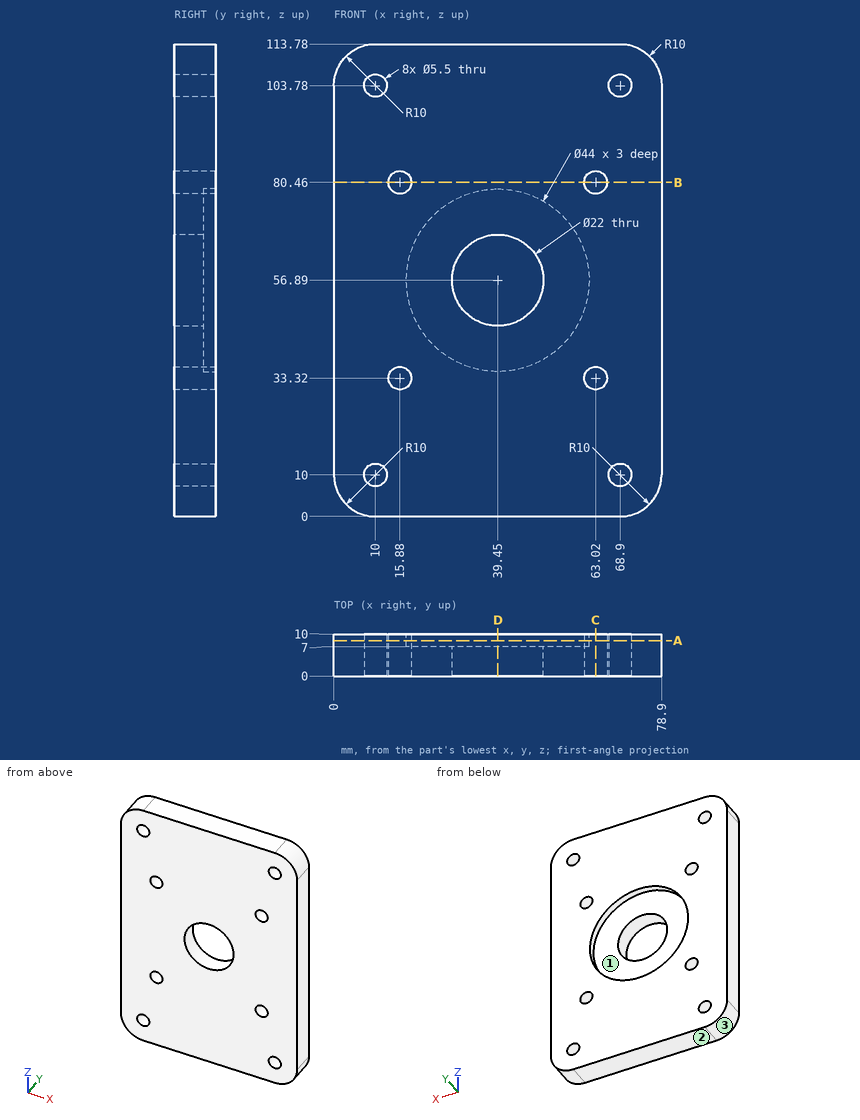
Job drawing, mm, ordinate dimensions from the low corner. One solid piece. Round coordinates to 2 decimals unless told otherwise and drop trailing zeros. Write each loop counter-clockwise with the first axis right and the second up, starting at its lowest first coordinate (ties: lowest second). Pieces come first, ordered by that corner, then holes.
1) Mould opens along X. For the marked faces 1, 2 and 3 say: +X half, -X half, draft (parallel to the pull), parting line (faces both ways), or undercut.
2) Band-saw the part on A-A, the plane y = 8.5. Give the number of separate pieces and of enclosed holes in the cut face, and give its area (3 significant figures).
3) Band-saw the part on B-B, the plane z = 80.46. List the corners of the cut face in (x, y).
4) Band-saw the part on C-C, the plane x = 63.02. List the corners of the cut face in (y, z).
5) Band-saw the part on D-D, the plane x = 39.45. List the corners of the cut face in (y, z), and give its area (3 significant figures).
6) Pin check, flat tips, straight feed: pin 1 (3.5 mm diameter, centred on x = 15.88, z = 80.46, fed in from +Y); pin 2 (12 mm diameter, centred on x = 29, z = 47, fed in from +Y). Stop position of each tip, or through.
7) Drill centre lines: probe 1 along X at (y, z) = (5, 103.78); probe 2 along X at (y, z) = (8, 80.46); probe 3 along Z at (x, y) = (69, 4.5). Where is each one in solid material? Low to high.
Ans:
1. face 1: undercut
1. face 2: draft
1. face 3: -X half
2. separate pieces: 1
2. enclosed holes: 9
2. area: 7,180 mm2
3. outline: (0, 0) - (13.13, 0) - (13.13, 10) - (0, 10) - close; (18.63, 0) - (60.27, 0) - (60.27, 10) - (18.63, 10) - close; (65.77, 0) - (78.9, 0) - (78.9, 10) - (65.77, 10) - close
4. outline: (0, 0) - (10, 0) - (10, 30.57) - (0, 30.57) - close; (0, 36.07) - (10, 36.07) - (10, 77.71) - (0, 77.71) - close; (0, 83.21) - (10, 83.21) - (10, 113.78) - (0, 113.78) - close
5. outline: (0, 0) - (10, 0) - (10, 34.89) - (7, 34.89) - (7, 45.89) - (0, 45.89) - close; (0, 67.89) - (7, 67.89) - (7, 78.89) - (10, 78.89) - (10, 113.78) - (0, 113.78) - close
5. area: 852 mm2
6. pin 1: passes through
6. pin 2: stops at y = 7
7. probe 1: x = 0 to 7.25, 12.75 to 66.15, 71.65 to 78.9
7. probe 2: x = 0 to 13.13, 18.63 to 60.27, 65.77 to 78.9
7. probe 3: z = 0 to 7.25, 12.75 to 101.03, 106.53 to 113.78
